Print and shaded views of the part. All mm, measured from the part's lowest x, y and z. A direction names the side the tool comes from. Coordinates: 2 decimals unless noted, no trailing zeros. Order: outer loops, then holes, each group sorted by start corner. A loop starts at its lowest first (then second) coordinate and runs counter-clockwise, first axis right, second up.
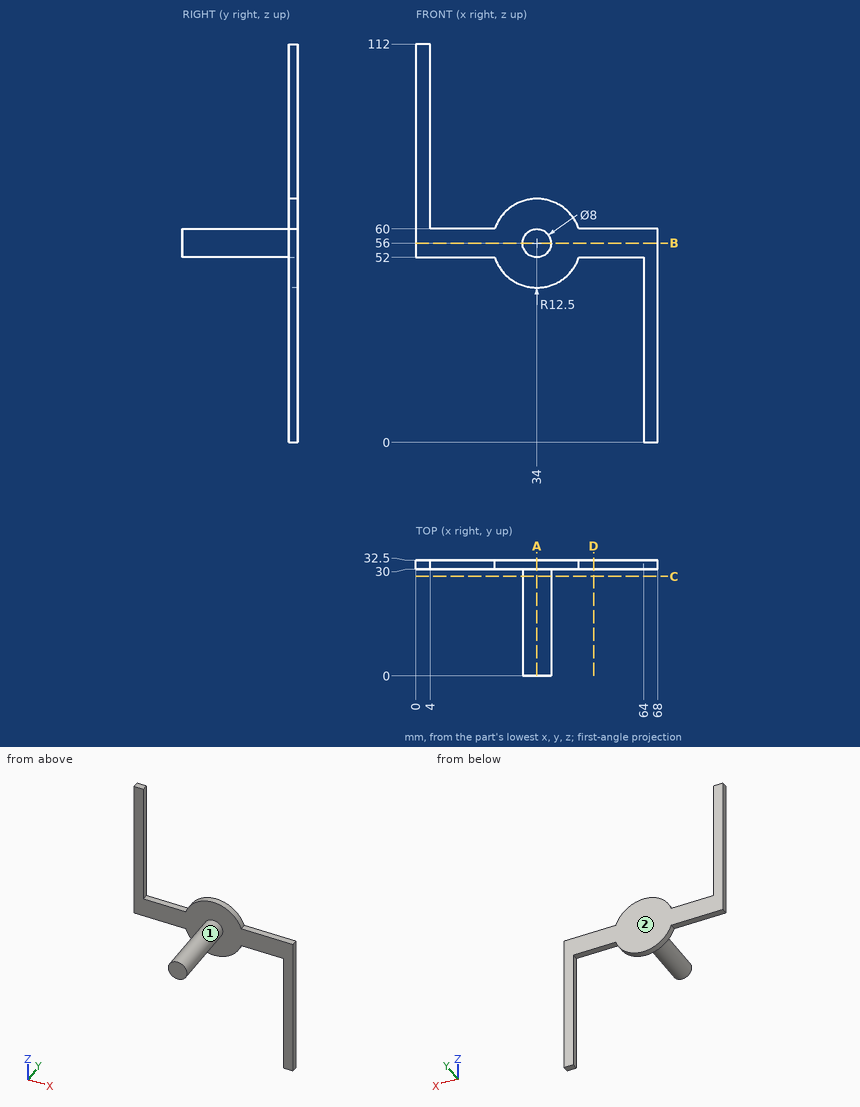
Q1. Cut at A-A, the plane x = 34. List the corners of the cut face in (y, z), plus the area to 4 significant figures.
Established:
outline: (0, 52) - (30, 52) - (30, 43.5) - (32.5, 43.5) - (32.5, 68.5) - (30, 68.5) - (30, 60) - (0, 60) - close
area: 302.5 mm2
Q2. Cut at C-C, the plane y = 28. List the corners of the cut face in (x, z), plus the area to 3 significant figures.
Established:
outline: circle Ø8 at (34, 56)
area: 50.3 mm2
Q3. Cut at B-B, the plane z = 56. List the corners of the cut face in (x, y).
Established:
outline: (0, 30) - (30, 30) - (30, 0) - (38, 0) - (38, 30) - (68, 30) - (68, 32.5) - (0, 32.5) - close
Q4. Which spindle directions (+Z, -Z, +X, -X, +Y, -Y) get a long thin tool onto all of the face, cutting with end or side? Do the marked faces 1 and 2. Say none if no direction does.
Established:
face 1: -Y
face 2: +Z, -Z, +X, -X, +Y
Q5. Probe line 1 (Y direction, x = 35, z = 62); line 2 (Z direction, x = 34.5, y = 7.5); line 3 (X direction, y = 31, z = 69.5). List the from-to ranges inside material, lowest first.
Established:
line 1: y = 30 to 32.5
line 2: z = 52.03 to 59.97
line 3: x = 0 to 4
Q6. Cut at D-D, the plane x = 50. List the corners of the cut face in (y, z).
Established:
outline: (30, 52) - (32.5, 52) - (32.5, 60) - (30, 60) - close
Q7. Drop flat-ended pins along their axis: P1, Ø3, axis at x = 6, y = 31, coming from the -Z side; P2, Ø0.8, axis at x = 62, y = 30.5, coming from the +Z side; P3, Ø1.2, axis at y = 30.5, z = 27, coming from the -X side; P4, Ø1, axis at x = 28.5, y = 28, coming from the +Z side. Give the stop position or say it passes through.
Established:
P1: stops at z = 52
P2: stops at z = 60
P3: stops at x = 64
P4: passes through
